from build123d import *

# Parameters (mm, degrees)
SKETCH1_R           = 4
BOSS_EXTRUDE1_DEPTH = 12
SKETCH2_R           = 2.25
CUT_EXTRUDE1_DEPTH  = 12


with BuildPart() as part:
    # Sketch1 → Boss-Extrude1 (new body)
    with BuildSketch(Plane(origin=(0, 0, 0), x_dir=(1, 0, 0), z_dir=(0, 1, 0))):
        with BuildLine():
            Line((-27.5, -10), (-27.5, -15))
            Line((-27.5, -15), (-14.5, -15))
            Line((-14.5, -15), (-12.366440747, -7.571072794))
            ThreePointArc((-12.366440747, -7.571072794), (0, -14.5), (12.366440747, -7.571072794))
            Line((12.366440747, -7.571072794), (14.5, -15))
            Line((14.5, -15), (27.5, -15))
            Line((27.5, -15), (27.5, -10))
            Line((27.5, -10), (16.942866484, -10))
            Line((16.942866484, -10), (14.5, 0))
            ThreePointArc((14.5, 0), (0, 14.5), (-14.5, 0))
            Line((-14.5, 0), (-16.942866484, -10))
            Line((-16.942866484, -10), (-27.5, -10))
        make_face()
        Circle(SKETCH1_R, mode=Mode.SUBTRACT)
    extrude(amount=BOSS_EXTRUDE1_DEPTH)

    # Sketch2 → Cut-Extrude1 (cut)
    with BuildSketch(Plane.XY.offset(15)):
        with Locations((-21, 6)):
            Circle(SKETCH2_R)
        with Locations((21, 6)):
            Circle(SKETCH2_R)
    extrude(amount=-CUT_EXTRUDE1_DEPTH, mode=Mode.SUBTRACT)


solid = part.part
Part model, mm, in its own coordinate system. A direction names the side the tool comes from. Coordinates: 2 decimals unless noted, no trailing zeros. Loops run counter-clockwise (first coordinate to the right, second up) from the corner with the lowest first, then second, coordinate; pieces in that order, holes last. Notation, with made-up numbers: (55, 64.5) - (106, 64.5) arc R37 cw to (106, 101.5) - close; hole circle Ø4 at (3.25, -22.75). An arc over 180 degrees is marked (long way). Write each question's results on one line, items separated by ' | '. Start each with the question number.
Q1. Which spindle directions (+Z, -Z, +X, -X, +Y, -Y) get a long thin tool onto all of the face, cutting with end or side? Do faces 4 (the flat face through (-23.3, 4.6, 10)), 5 (the flat face through (23.5, 5.9, 10)), 6 (the flat face through (0, 12, 7)). Say none if no direction does.
Q2. Slice it at B-B on y = 5. Give the cut face in (x, z), and give its area (3 significant figures).
Q3. Two-plate mould, pull along X, no slides. Class faces 1 (the flat face through (0, 0, 7)), 2 (the cylindrical face through (0.319, 5.916, -14.496)), 3 (the flat face through (-13.45, 5.92, 11.34)): +X half, -X half, draft (parallel to the pull), parting line (faces both ways), or undercut.
Q4. Slice it at A-A on x = -21. Give the cut face in (y, z), and give its area (3 significant figures).
Q5. Probe line 1 along Y through (x, z) = (-21, 12.1); line 2 along Z through (x, y) = (0, 8.25); line 3 along Z through (x, y) = (-18, 10.5). List the from-to ranges inside material, lowest first.
Q6. Drop flat-ended pins along their axis: pin 1 Ø4 at (x, y) = (13.5, 3.5) entering from -Z; pin 2 Ø4 at (x, y) = (-10, 5) entering from -Z; pin 3 Ø2.5 at (x, y) = (21, 6) entering from -Z; pin 4 Ø5 at (x, y) = (-21, 6) entering from -Z. Give the stop position or say it passes through.
Q7. Slice it at D-D on y = 9.75. Give the cut face in (x, z).
Q8. Slice it at C-C on z = 8.75. Give the cut face in (x, y), and give its area (3 significant figures).
Answer:
1) face 4: -Z, -X, +Y, -Y | face 5: -Z, +X, +Y, -Y | face 6: +Z, -Z, +X, -X, +Y
2) outline: (-27.5, 10) - (-23.02, 10) - (-23.02, 15) - (-27.5, 15) - close; (-18.98, 10) - (-16.94, 10) - (-14.5, 0) arc R14.5 ccw to (14.5, 0) - (16.94, 10) - (18.98, 10) - (18.98, 15) - (14.5, 15) - (12.37, 7.57) arc R14.5 ccw to (-12.37, 7.57) - (-14.5, 15) - (-18.98, 15) - close; (23.02, 10) - (27.5, 10) - (27.5, 15) - (23.02, 15) - close; hole circle Ø8 at (0, 0) | area: 751 mm2
3) face 1: draft | face 2: parting line | face 3: undercut
4) outline: (0, 10) - (3.75, 10) - (3.75, 15) - (0, 15) - close; (8.25, 10) - (12, 10) - (12, 15) - (8.25, 15) - close | area: 37.5 mm2
5) line 1: y = 0 to 3.75, 8.25 to 12 | line 2: z = -14.5 to -4, 4 to 14.5 | line 3: z = 10 to 15
6) pin 1: stops at z = -8.83 | pin 2: stops at z = -12.09 | pin 3: passes through | pin 4: stops at z = 10
7) outline: (-27.5, 10) - (-16.94, 10) - (-14.5, 0) arc R14.5 ccw to (14.5, 0) - (16.94, 10) - (27.5, 10) - (27.5, 15) - (14.5, 15) - (12.37, 7.57) arc R14.5 ccw to (-12.37, 7.57) - (-14.5, 15) - (-27.5, 15) - close; hole circle Ø8 at (0, 0)
8) outline: (-16.64, 0) - (-12.71, 0) - (-12.71, 12) - (-16.64, 12) - close; (-11.56, 0) - (11.56, 0) - (11.56, 12) - (-11.56, 12) - close; (12.71, 0) - (16.64, 0) - (16.64, 12) - (12.71, 12) - close | area: 372 mm2
